```python
from build123d import *

# Parameters (mm, degrees)
F0_R     = 12.5
F1_DEPTH = 25
F2_R     = 25
F2_R_2   = 2.5
F3_DEPTH = 5
F4_R     = 3


with BuildPart() as f1:
    # F0 (on Front) → F1 (new body, symmetric)
    with BuildSketch(Plane.XZ):
        Circle(F0_R)
    extrude(amount=F1_DEPTH, both=True)

    # F2 (on Front) → F3 (join, symmetric)
    with BuildSketch(Plane.XZ):
        Circle(F2_R)
        with Locations((-8.6776747824, -18.019377358)):
            Circle(F2_R_2, mode=Mode.SUBTRACT)
        with Locations((-15.6366296494, -12.4697960372)):
            Circle(F2_R_2, mode=Mode.SUBTRACT)
        with Locations((-19.4985582436, -4.4504186791)):
            Circle(F2_R_2, mode=Mode.SUBTRACT)
        with Locations((0, -20)):
            Circle(F2_R_2, mode=Mode.SUBTRACT)
        with Locations((8.6776747824, -18.019377358)):
            Circle(F2_R_2, mode=Mode.SUBTRACT)
        with Locations((15.6366296494, -12.4697960372)):
            Circle(F2_R_2, mode=Mode.SUBTRACT)
        with Locations((19.4985582436, -4.4504186791)):
            Circle(F2_R_2, mode=Mode.SUBTRACT)
        with Locations((-19.4985582436, 4.4504186791)):
            Circle(F2_R_2, mode=Mode.SUBTRACT)
        with Locations((-15.6366296494, 12.4697960372)):
            Circle(F2_R_2, mode=Mode.SUBTRACT)
        with Locations((-8.6776747824, 18.019377358)):
            Circle(F2_R_2, mode=Mode.SUBTRACT)
        with Locations((19.4985582436, 4.4504186791)):
            Circle(F2_R_2, mode=Mode.SUBTRACT)
        with Locations((15.6366296494, 12.4697960372)):
            Circle(F2_R_2, mode=Mode.SUBTRACT)
        with Locations((8.6776747824, 18.019377358)):
            Circle(F2_R_2, mode=Mode.SUBTRACT)
        with Locations((0, 20)):
            Circle(F2_R_2, mode=Mode.SUBTRACT)
    extrude(amount=F3_DEPTH, both=True)

    # F4
    f4_edges = [f1.edges().sort_by_distance(p)[0] for p in [
        (-12.5, 5, 0),
        (-12.5, -5, 0),
    ]]
    fillet(f4_edges, radius=F4_R)


solid = f1.part
```
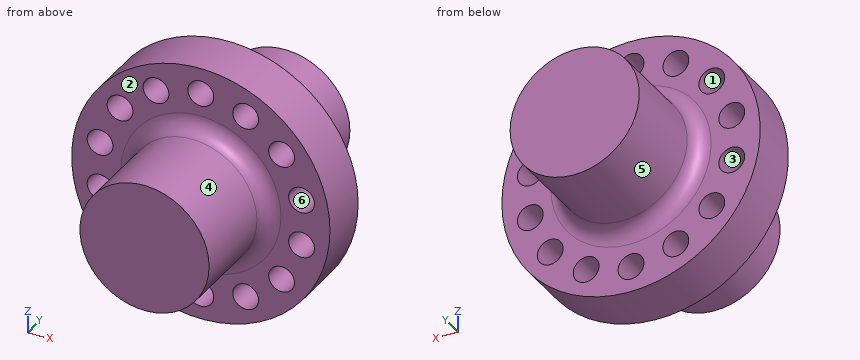
Here's how the part is built. I have some questions about the finished solid (model axes, mm). Face numbers are marked on the shaded views. A direction names the side the tool comes from. Give positions to 0.01 mm unless a question says otherwise; leave off trailing zeros. Write each loop counter-clockwise with the first axis right and the second up, starting at its lowest first coordinate (ties: lowest second). Pieces come first, ordered by that corner, then holes. Notation, with made-up numbers: (33.25, 59.25) -> (42.25, 59.25) arc R31 ccw to (42.25, 98.25) -> close; hole circle Ø2 at (-31.5, 19). An arc over 180 degrees is marked (long way). Write each question's results on one line, items separated by ' | '.
Item 1: We'd pull the mould along X, two halves only. Please class the marked faces 1, 2, 3 and 4: pulls with the +X half, pulls with the -X half, needs draft (parallel to the pull), parting line crosses it, or undercut.
Output:
face 1: undercut | face 2: needs draft | face 3: undercut | face 4: parting line crosses it
Item 2: Suppose I cut it at D-D on y = -17. Write out the boundary of the cut face in (x, z), plus the area to 3 significant figures.
Output:
outline: circle Ø25 at (0, 0) | area: 491 mm^2
Item 3: On a 3-axis mill with a long thin cutter (end or side, diameter ignored), from which of +Z, -Z, +X, -X, +Y, -Y can I reach the whole of each face in a straight line? I mean the marked faces 5 and 6. Say none if no direction works.
Output:
face 5: +Y | face 6: +Y, -Y
Item 4: Suppose I cut it at C-C on x = -19.5. Write out the boundary of the cut face in (y, z), plus the area to 3 significant figures.
Output:
outline: (-5, -15.64) -> (5, -15.64) -> (5, -6.95) -> (-5, -6.95) -> close; (-5, -1.95) -> (5, -1.95) -> (5, 1.95) -> (-5, 1.95) -> close; (-5, 6.95) -> (5, 6.95) -> (5, 15.64) -> (-5, 15.64) -> close | area: 213 mm^2
Item 5: Suppose I cut it at A-A on x = 0. Write out the boundary of the cut face in (y, z), plus the area to 3 significant figures.
Output:
outline: (-25, -12.5) -> (-8, -12.5) arc R3 cw to (-5, -15.5) -> (-5, -17.5) -> (5, -17.5) -> (5, -15.5) arc R3 cw to (8, -12.5) -> (25, -12.5) -> (25, 12.5) -> (8, 12.5) arc R3 cw to (5, 15.5) -> (5, 17.5) -> (-5, 17.5) -> (-5, 15.5) arc R3 cw to (-8, 12.5) -> (-25, 12.5) -> close; (-5, -25) -> (5, -25) -> (5, -22.5) -> (-5, -22.5) -> close; (-5, 22.5) -> (5, 22.5) -> (5, 25) -> (-5, 25) -> close | area: 1,410 mm^2
Item 6: Suppose I cut it at B-B on z = 0. Write out the boundary of the cut face in (x, y).
Output:
outline: (-25, -5) -> (-15.5, -5) arc R3 cw to (-12.5, -8) -> (-12.5, -25) -> (12.5, -25) -> (12.5, -8) arc R3 cw to (15.5, -5) -> (25, -5) -> (25, 5) -> (15.5, 5) arc R3 cw to (12.5, 8) -> (12.5, 25) -> (-12.5, 25) -> (-12.5, 8) arc R3 cw to (-15.5, 5) -> (-25, 5) -> close
Item 7: For pin 1 Ø8 at (x, z) = (-15.64, 12.47) entering from -Y; pin 2 Ø3 at (y, z) = (-10.5, -5.5) entering from -X; pin 3 Ø8 at (x, z) = (8.68, -18.02) entering from +Y; pin 4 Ø4 at (x, z) = (19.5, -4.45) entering from +Y, each with a flat end and sliding along its axis, tell me the tip position at first contact or that it passes through.
Output:
pin 1: stops at y = -5 | pin 2: stops at x = -11.84 | pin 3: stops at y = 5 | pin 4: passes through
Item 8: If I drill on L1, parallel to X at y = -1, z = -18.5; L2, parallel to Y at x = 3.5, z = 18.5; L3, parallel to Z at x = 7.5, y = 14.5, over which ranges is the centre line in solid material (lowest first)?
Output:
L1: x = -16.82 to -11.13, -6.22 to -2, 2 to 6.22, 11.13 to 16.82 | L2: y = -5 to 5 | L3: z = -10 to 10
